from build123d import *

# Parameters (mm, degrees)
F1_DEPTH = 5
F2_R     = 2


with BuildPart() as f1:
    # F0 (on Top) → F1 (new body)
    with BuildSketch(Plane.XY):
        with BuildLine():
            ThreePointArc((-30, -40), (0, -31.961524), (30, -40))
            ThreePointArc((30, -40), (0, 50), (-30, -40))
        make_face()
    extrude(amount=F1_DEPTH)

    # F2
    f2_edges = [f1.edges().sort_by_distance(p)[0] for p in [
        (0, -31.961524, 5),
        (0, 50, 5),
        (0, -31.961524, 0),
        (0, 50, 0),
    ]]
    fillet(f2_edges, radius=F2_R)


solid = f1.part
CAD build for the part. Positions are in the model's coordinates, mm. Coordinates: 2 decimals unless noted, no trailing zeros. Order: outer loops, then holes, each group sorted by start corner. A loop starts at its lowest first (then second) coordinate and runs counter-clockwise, first axis right, second up.
Item 1: Two-plate mould, pull along X, no slides. Class faces 1 (the face through (-0.44, -31.963, 2.493)), 2 (the face through (-1, 6, 5)), 3 (the face through (1.75, 49.97, 2.49)): +X half, -X half, draft (parallel to the pull), parting line (faces both ways), or undercut.
Check sheet entries:
face 1: undercut
face 2: draft
face 3: parting line
Item 2: Drill centre lines: L1, parallel to Z at x = -39, y = -29.5; L2, parallel to Y at x = -26.5, z = 0.9; L3, parallel to Y at x = 10, z = 3.15. Where is each one in solid material? Low to high.
Check sheet entries:
L1: z = 0.21 to 4.79
L2: y = -37.76 to 42.01
L3: y = -32.8 to 48.98
Item 3: Band-saw the part on A-A on x = 0. List the corners of the cut face in (y, z), plus the area to 3 significant figures.
Check sheet entries:
outline: (-31.96, 2) arc R2 ccw to (-29.96, 0) - (48, 0) arc R2 ccw to (50, 2) - (50, 3) arc R2 ccw to (48, 5) - (-29.96, 5) arc R2 ccw to (-31.96, 3) - close
area: 406 mm2
Item 4: Pin check, flat tips, straight feed: pin 1 Ø1.5 at (y, z) = (-21.5, 1.5) entering from -X; pin 2 Ø1 at (x, z) = (-11, 4.5) entering from +Y. Stop position of each tip, or through.
Check sheet entries:
pin 1: stops at x = -45.45
pin 2: stops at y = 48.52
Item 5: Band-saw the part on B-B on z = 4.15. List the corners of the cut face in (x, y), plus the area to 3 significant figures.
Check sheet entries:
outline: (-29.97, -39.56) arc R60.36 cw to (29.97, -39.56) arc R49.64 ccw (long way) to start
area: 7,010 mm2
